Work out the finished part from the listing and answer in its coordinate system (mm). A direction names the side the tool comes from. Give positions to 0.01 mm unless a question says otherwise; leave off trailing zeros. Order: outer loops, then holes, each group sorted by start corner. A loop starts at its lowest first (then second) coordinate and runs counter-clockwise, first axis right, second up. Notation, with made-up numbers: M 74,-28 L 83,-28 A21 cw 83,-21 Z; hole C -7,-26 d3. An arc over 180 degrees is marked long. One line per item, written item: value.
from build123d import *

# Parameters (mm, degrees)
SKETCH_1_W                 = 45
SKETCH_1_H                 = 17.5
EXTRUDE_2_DEPTH            = 5.9
CUT_EXTRUDE_1_DEPTH        = 10
CUT_EXTRUDE_1_DEPTH_BACK   = 2.4
FILLET_1_R                 = 1
FILLET_2_R                 = 1
FILLET_5_R                 = 1
FILLET_6_R                 = 1
FILLET_7_R                 = 0.5
SKETCH_5_R                 = 0.5
CUT_EXTRUDE_2_DEPTH        = 4.5
CHAMFER_1_SIZE             = 0.1
CHAMFER_1_OF_MIRROR_1_SIZE = 0.1
SKETCH_20_W                = 5
SKETCH_20_H                = 17.5
EXTRUDE_3_DEPTH            = 1.4
FILLET_8_R                 = 0.5
SKETCH_21_R                = 0.5
CUT_EXTRUDE_3_DEPTH        = 11


# Read off the part's stored shape, not the designer's step: 镜向2
with BuildPart() as part:
    # 草图1 → 凸台-拉伸2 (new body)
    with BuildSketch(Plane(origin=(0, 0, 0), x_dir=(1, 0, 0), z_dir=(0, 1, 0))):
        with Locations((2.5, 0)):
            Rectangle(SKETCH_1_W, SKETCH_1_H)
    extrude(amount=EXTRUDE_2_DEPTH)

    # 草图3 → 切除-拉伸1 (cut, two sides: drawn at the far end of the back side and taken through both)
    with BuildSketch(Plane(origin=(0, 3.8, 0), x_dir=(1, 0, 0), z_dir=(0, 1, 0)).offset(-CUT_EXTRUDE_1_DEPTH_BACK)):
        with BuildLine():
            Line((-17, -6.5), (-17, -7))
            ThreePointArc((-17, -7), (-16.5, -7.5), (-16, -7))
            Line((-16, -7), (15.751729614, -7))
            ThreePointArc((15.751729614, -7), (16.605283005, -7.353553391), (16.251729614, -6.5))
            Line((16.251729614, -6.5), (16.251729614, 6.5))
            ThreePointArc((16.251729614, 6.5), (16.605283005, 7.353553391), (15.751729614, 7))
            Line((15.751729614, 7), (-16, 7))
            ThreePointArc((-16, 7), (-16.5, 7.5), (-17, 7))
            Line((-17, 7), (-17, 6.5))
            Line((-17, 6.5), (-17, 6))
            Line((-17, 6), (-20, 6))
            Line((-20, 6), (-20, -6))
            Line((-20, -6), (-17, -6))
            Line((-17, -6), (-17, -6.5))
        make_face()
    extrude(amount=CUT_EXTRUDE_1_DEPTH + CUT_EXTRUDE_1_DEPTH_BACK, mode=Mode.SUBTRACT)

    # 圆角1
    fillet_1_edges = [part.edges().sort_by_distance(p)[0] for p in [
        (16.251729614, 3.65, -6.5),
    ]]
    fillet(fillet_1_edges, radius=FILLET_1_R)

    # 圆角2
    fillet_2_edges = [part.edges().sort_by_distance(p)[0] for p in [
        (15.751729614, 3.65, -7),
    ]]
    fillet(fillet_2_edges, radius=FILLET_2_R)

    # 圆角5
    fillet_5_edges = [part.edges().sort_by_distance(p)[0] for p in [
        (-16, 3.65, 7),
        (-16, 3.65, -7),
    ]]
    fillet(fillet_5_edges, radius=FILLET_5_R)

    # 圆角6
    fillet_6_edges = [part.edges().sort_by_distance(p)[0] for p in [
        (15.751729614, 3.65, 7),
        (16.251729614, 3.65, 6.5),
    ]]
    fillet(fillet_6_edges, radius=FILLET_6_R)

    # 圆角7
    fillet_7_edges = [part.edges().sort_by_distance(p)[0] for p in [
        (2.5, 0, -8.75),
        (2.5, 0, 8.75),
    ]]
    fillet(fillet_7_edges, radius=FILLET_7_R)

    # 草图5 → 切除-拉伸2 (cut)
    with BuildSketch(Plane(origin=(0, 5.9, 0), x_dir=(1, 0, 0), z_dir=(0, 1, 0))):
        with Locations(Location((-18.5, 7.375, 0), (0, 0, 270))):
            Circle(SKETCH_5_R)
    cut_extrude_2 = extrude(amount=-CUT_EXTRUDE_2_DEPTH, mode=Mode.SUBTRACT)

    # 倒角1
    chamfer_1_edges = [part.edges().sort_by_distance(p)[0] for p in [
        (-18.5, 5.9, -7.875),
    ]]
    chamfer(chamfer_1_edges, length=CHAMFER_1_SIZE)

    # 镜向1: 切除-拉伸2 across plane
    add(cut_extrude_2.mirror(Plane.XY), mode=Mode.SUBTRACT)

    # 倒角1 of 镜向1
    chamfer_1_of_mirror_1_edges = [part.edges().sort_by_distance(p)[0] for p in [
        (-18.5, 5.9, 7.875),
    ]]
    chamfer(chamfer_1_of_mirror_1_edges, length=CHAMFER_1_OF_MIRROR_1_SIZE)

    # 镜向2 outline → 镜向2 (revolve, cut)
    with BuildSketch(Plane(origin=(18.5, 0, -7.375), x_dir=(1, 0, 0), z_dir=(0, 0, 1))):
        Polygon((0, 5.9), (0, 1.4), (0.5, 1.4), (0.5, 5.8), (0.6, 5.9), align=None)
    revolve(axis=Axis((18.5, 0, -7.375), (0, 1, 0)), mode=Mode.SUBTRACT)

    # Mirror 2 2 outline → Mirror 2 2 (revolve, cut)
    with BuildSketch(Plane(origin=(18.5, 0, 7.375), x_dir=(1, 0, 0), z_dir=(0, 0, 1))):
        Polygon((0, 5.9), (0, 1.4), (0.5, 1.4), (0.5, 5.8), (0.6, 5.9), align=None)
    revolve(axis=Axis((18.5, 0, 7.375), (0, 1, 0)), mode=Mode.SUBTRACT)

    # 草图20 → 凸台-拉伸3 (add)
    with BuildSketch(Plane(origin=(0, 5.9, 0), x_dir=(1, 0, 0), z_dir=(0, 1, 0))):
        with Locations((22.5, 0)):
            Rectangle(SKETCH_20_W, SKETCH_20_H)
    extrude(amount=EXTRUDE_3_DEPTH)

    # 圆角8
    fillet_8_edges = [part.edges().sort_by_distance(p)[0] for p in [
        (22.5, 7.3, 8.75),
        (22.5, 7.3, -8.75),
    ]]
    fillet(fillet_8_edges, radius=FILLET_8_R)

    # 草图21 → 切除-拉伸3 (cut)
    with BuildSketch(Plane(origin=(0, 0, 0), x_dir=(1, 0, 0), z_dir=(0, 1, 0))):
        with Locations(Location((22.5, 0, 0), (0, 0, 270))):
            Circle(SKETCH_21_R)
    extrude(amount=CUT_EXTRUDE_3_DEPTH, mode=Mode.SUBTRACT)


solid = part.part
(1) Section B-B, the plane z = 0 is taken. Give the vertices of the cut face in (x, y).
Findings:
outline: M -20,0 L 22,0 L 22,7.3 L 20,7.3 L 20,5.9 L 16.25,5.9 L 16.25,1.4 L -20,1.4 Z; M 23,0 L 25,0 L 25,7.3 L 23,7.3 Z
(2) Determine the mould class of faces 4 (the flat face through (2, 4, 8.75)), 5 (the flat face through (0, 4, 7)), 6 (the flat face through (-20, 1, 0)) for opening direction Z: pulls with the +Z half, pulls with the -Z half, needs draft (parallel to the pull), parting line crosses it, or undercut.
Findings:
face 4: pulls with the +Z half
face 5: undercut
face 6: needs draft
(3) Find the intervals of material crossed by probe 1 along X at (y, z) = (3, 7.75); probe 2 along X at (y, z) = (3.75, 0); probe 3 along Z at (x, y) = (-7, 2.25), in increasing order. Write a range as from..to.
Findings:
probe 1: x = -20..-18.83, -18.17..18.17, 18.83..25
probe 2: x = 16.25..22, 23..25
probe 3: z = -8.75..-7, 7..8.75
(4) Section C-C, the plane x = -5.5 is taken. Give the vertices of the cut face in (y, z), then the cut area to 3 significant figures.
Findings:
outline: M 0,-8.25 A0.5 ccw 0.5,-8.75 L 5.9,-8.75 L 5.9,-7 L 1.4,-7 L 1.4,7 L 5.9,7 L 5.9,8.75 L 0.5,8.75 A0.5 ccw 0,8.25 Z
area: 40.1 mm^2
(5) Section D-D, the plane y = 5.25 is taken. Give the vertices of the cut face in (x, z) (3 decimals), then the cut area to 3 significant figures.
Findings:
outline: M -20,-8.75 L 25,-8.75 L 25,8.75 L -20,8.75 L -20,6 L -17,6 L -17,7 A0.5 cw -16.127,7.333 A1 ccw -15.382,7 L 15.134,7 A1 ccw 15.879,7.333 A0.5 cw long 16.585,6.627 A1 ccw 16.252,5.882 L 16.252,-5.882 A1 ccw 16.585,-6.627 A0.5 cw long 15.879,-7.333 A1 ccw 15.134,-7 L -15.382,-7 A1 ccw -16.127,-7.333 A0.5 cw -17,-7 L -17,-6 L -20,-6 Z; hole C -18.5,-7.375 d1; hole C -18.5,7.375 d1; hole C 18.5,-7.375 d1; hole C 18.5,7.375 d1; hole C 22.5,0 d1
area: 280 mm^2
(6) Given P1, Ø4, axis at x = -8, z = 0.5, coming from the +Y side; P2, Ø0.5, axis at x = -18.5, z = -7, coming from the +Y side; P3, Ø1.5, axis at y = 6, z = -3, coming from the -X side; P4, Ø3, axis at x = 19.5, z = -7, coming from the +Y side, each flat-ended and moving along its own axis, determine where each tip first touches the part or whether it passes through.
Findings:
P1: stops at y = 1.4
P2: stops at y = 5.9
P3: stops at x = 16.25
P4: stops at y = 7.3
(7) Section A-A, the plane x = 22.5 is taken. Give the vertices of the cut face in (y, z), then the cut area to 3 significant figures.
Findings:
outline: M 0,-8.25 A0.5 ccw 0.5,-8.75 L 6.8,-8.75 A0.5 ccw 7.3,-8.25 L 7.3,-0.5 L 0,-0.5 Z; M 0,0.5 L 7.3,0.5 L 7.3,8.25 A0.5 ccw 6.8,8.75 L 0.5,8.75 A0.5 ccw 0,8.25 Z
area: 120 mm^2
(8) Which of the six approach directions +Z, -Z, +X, -X, +Y, -Y give full straight-line access (tool end or side, diameter ignored) to faces 1 (the flat face through (-18, 4, -6)), 2 (the flat face through (-17, 3.6, -6.5)), 3 (the flat face through (20, 7, 0))?
Findings:
face 1: -X, +Y
face 2: +Y
face 3: +Z, -Z, -X, +Y
